Part model, mm, in its own coordinate system. Face numbers are marked on the shaded views. A direction names the side the tool comes from. Round coordinates to 2 decimals unless told otherwise and drop trailing zeros. Write each loop counter-clockwise with the first axis right and the second up, starting at its lowest first coordinate (ties: lowest second). Pieces come first, ordered by that corner, then holes. Notation, with made-up numbers: (58.5, 89) -> (103.5, 89) arc R30 ccw to (103.5, 120) -> close; hole circle Ø3 at (-3.75, -33.75). An arc over 180 degrees is marked (long way). Use CSV: the item, a comma, the result in double quotes. Start each with the question number.
(1) Saw through at A-A (x = 22.5). Give the cut face in (y, z).
(2) Which spindle directions (+Z, -Z, +X, -X, +Y, -Y) get a long thin tool onto all of the face, cutting with end or side? Do the marked faces 4 and 5. Say none if no direction does.
(3) Saw through at C-C (z = 7.5). Count the separate pieces of the cut face and the enclosed holes in it, plus the area to 3 significant figures.
(4) Probe line 1 (Y direction, x = -14.5, z = 1.5); line 2 (Y direction, x = -17, z = 12.25); line 3 (X direction, y = 128.5, z = 9.75). List the from-to ranges inside material, lowest first. Write a range as [from, to].
(5) Saw through at B-B (y = 22). Give the cut face in (x, z), plus the area to 3 significant figures.
(6) Drop flat-ended pins along their axis: pin 1 (4 mm diameter, centred on y = 35, z = 9.5, fed in from -X); pin 2 (3 mm diameter, centred on x = 9.525, y = 79.375, fed in from +Z); pin 3 (1.5 mm diameter, centred on y = 120, z = 7.5, fed in from -X); pin 4 (3 mm diameter, centred on x = 65, z = 4.5, fed in from +Y). Give the stop position or say it passes through.
(7) Two-plate mould, pull along Y, no slides. Class the marked faces 1, 2 and 3: released by +Y, released by -Y, zero draft, split by the parting line, or undercut.
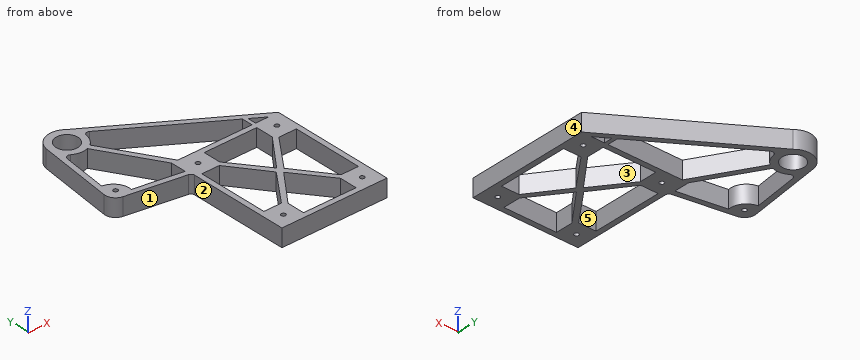
```python
from build123d import *

# Parameters (mm, degrees)
SKETCH1_R           = 7.9375
BOSS_EXTRUDE1_DEPTH = 12.7
CUT_EXTRUDE1_DEPTH  = 12.7
SKETCH3_R           = 1.5875
CUT_EXTRUDE2_DEPTH  = 12.7
CUT_EXTRUDE3_DEPTH  = 12.7
FILLET1_R           = 2.54
BOSS_EXTRUDE2_DEPTH = 12.7
SKETCH6_R           = 1.5875
CUT_EXTRUDE4_DEPTH  = 12.7
FILLET2_R           = 7.62
FILLET3_R           = 2.54


with BuildPart() as part:
    # Sketch1 → Boss-Extrude1 (new body)
    with BuildSketch(Plane.XY):
        with BuildLine():
            Line((0, 0), (76.2, 0))
            Line((76.2, 0), (76.2, 88.9))
            Line((76.2, 88.9), (-21.190795437, 151.964199177))
            ThreePointArc((-21.190795437, 151.964199177), (-33.829972343, 154.632550249), (-42.545, 145.0975))
            Line((-42.545, 145.0975), (-50.8, 82.136361391))
            Line((-50.8, 82.136361391), (0, 73.66))
            Line((0, 73.66), (0, 0))
        make_face()
        with Locations((-29.845, 142.24)):
            Circle(SKETCH1_R, mode=Mode.SUBTRACT)
    extrude(amount=BOSS_EXTRUDE1_DEPTH)

    # Sketch2 → Cut-Extrude1 (cut)
    with BuildSketch(Plane.XY.offset(12.7)):
        Polygon((19.05, 3.81), (57.15, 3.81), (57.15, 16.51), (38.1, 41.5925), (19.05, 16.51), align=None)
        Polygon((3.81, 19.05), (16.51, 19.05), (35.2425, 44.45), (16.51, 69.85), (3.81, 69.85), align=None)
        Polygon((19.05, 85.09), (19.05, 72.39), (38.1, 47.3075), (57.15, 72.39), (57.15, 85.09), align=None)
        Polygon((72.39, 69.85), (59.69, 69.85), (40.9575, 44.45), (59.69, 19.05), (72.39, 19.05), align=None)
    extrude(amount=-CUT_EXTRUDE1_DEPTH, mode=Mode.SUBTRACT)

    # Sketch3 → Cut-Extrude2 (cut)
    with BuildSketch(Plane.XY.offset(12.7)):
        with Locations((66.675, 79.375)):
            Circle(SKETCH3_R)
        with Locations((9.525, 79.375)):
            Circle(SKETCH3_R)
        with Locations((9.525, 9.525)):
            Circle(SKETCH3_R)
        with Locations((66.675, 9.525)):
            Circle(SKETCH3_R)
    extrude(amount=-CUT_EXTRUDE2_DEPTH, mode=Mode.SUBTRACT)

    # Sketch4 → Cut-Extrude3 (cut)
    with BuildSketch(Plane.XY.offset(12.7)):
        with BuildLine():
            Line((69.190325437, 88.9), (-17.449031417, 145.002238745))
            ThreePointArc((-17.449031417, 145.002238745), (-17.963027163, 137.755725085), (-22.364956463, 131.976523558))
            Line((-22.364956463, 131.976523558), (3.158582938, 88.9))
            Line((3.158582938, 88.9), (69.190325437, 88.9))
        make_face()
        with BuildLine():
            Line((-40.065465421, 134.701294104), (-45.058154169, 96.621903635))
            ThreePointArc((-45.058154169, 96.621903635), (-37.359379788, 92.092328445), (-35.269920717, 83.407724876))
            Line((-35.269920717, 83.407724876), (-1.27, 77.734582843))
            Line((-1.27, 77.734582843), (-1.27, 88.9))
            Line((-1.27, 88.9), (-25.751473381, 130.217810523))
            ThreePointArc((-25.751473381, 130.217810523), (-33.641083643, 130.12060443), (-40.065465421, 134.701294104))
        make_face()
    extrude(amount=-CUT_EXTRUDE3_DEPTH, mode=Mode.SUBTRACT)

    # Fillet1
    fillet1_edges = [part.edges().sort_by_distance(p)[0] for p in [
        (-40.065465421, 134.701294104, 6.35),
        (-17.449031417, 145.002238745, 6.35),
    ]]
    fillet(fillet1_edges, radius=FILLET1_R)

    # Sketch5 → Boss-Extrude2 (add)
    with BuildSketch(Plane.XY.offset(12.7)):
        Polygon((57.125325437, 88.9), (59.665325437, 88.9), (59.665325437, 95.06779537), (57.125325437, 96.712540802), align=None)
    extrude(amount=-BOSS_EXTRUDE2_DEPTH)

    # Sketch6 → Cut-Extrude4 (cut)
    with BuildSketch(Plane.XY.offset(12.7)):
        with Locations((-42.288108338, 88.441435979)):
            Circle(SKETCH6_R)
    extrude(amount=-CUT_EXTRUDE4_DEPTH, mode=Mode.SUBTRACT)

    # Fillet2
    fillet2_edges = [part.edges().sort_by_distance(p)[0] for p in [
        (-50.8, 82.136361391, 6.35),
    ]]
    fillet(fillet2_edges, radius=FILLET2_R)

    # Fillet3
    fillet3_edges = [part.edges().sort_by_distance(p)[0] for p in [
        (0, 73.66, 6.35),
    ]]
    fillet(fillet3_edges, radius=FILLET3_R)


solid = part.part
```
Answers:
1,outline,"(0, 0) -> (3.81, 0) -> (3.81, 12.7) -> (0, 12.7) -> close; (21.05, 0) -> (27.17, 0) -> (27.17, 12.7) -> (21.05, 12.7) -> close; (61.73, 0) -> (67.85, 0) -> (67.85, 12.7) -> (61.73, 12.7) -> close; (85.09, 0) -> (88.9, 0) -> (88.9, 12.7) -> (85.09, 12.7) -> close; (119.13, 0) -> (123.67, 0) -> (123.67, 12.7) -> (119.13, 12.7) -> close"
2,face 4,"+Z, -Z, +X, +Y, -Y"
2,face 5,"+Z, -Z"
3,separate pieces,"1"
3,enclosed holes,"13"
3,area,"4,020 mm²"
4,line 1,"y = [76.08, 79.94], [111.23, 118.7], [142.75, 147.63]"
4,line 2,"y = [76.5, 80.36], [115.45, 122.92], [141.38, 149.25]"
4,line 3,"x = [-44.72, -40.88], [-24.73, -20.31], [8.04, 15.05]"
5,outline,"(0, 0) -> (3.81, 0) -> (3.81, 12.7) -> (0, 12.7) -> close; (18.69, 0) -> (23.22, 0) -> (23.22, 12.7) -> (18.69, 12.7) -> close; (52.98, 0) -> (57.51, 0) -> (57.51, 12.7) -> (52.98, 12.7) -> close; (72.39, 0) -> (76.2, 0) -> (76.2, 12.7) -> (72.39, 12.7) -> close"
5,area,"212 mm²"
6,pin 1,"stops at x = 0"
6,pin 2,"passes through"
6,pin 3,"stops at x = -45.93"
6,pin 4,"stops at y = 97.12"
7,face 1,"released by -Y"
7,face 2,"zero draft"
7,face 3,"undercut"
